Design review of the part shown in the three views and the two pictorial views. Dimensions are in mm from the part's minimum x, y and z. Coordinates: 2 decimals unless noted, no trailing zeros. Loops run counter-clockwise (first coordinate to the right, second up) from the corner with the lowest first, then second, coordinate; pieces in that order, holes last. Notation, with made-up numbers: M 48,18.25 L 90,18.25 A23 ccw 90,34.25 Z; hole C -6.75,-16 d8. An arc over 180 degrees is marked long. Use CSV: the item, a comma, the result in double quotes. Start each with the question number.
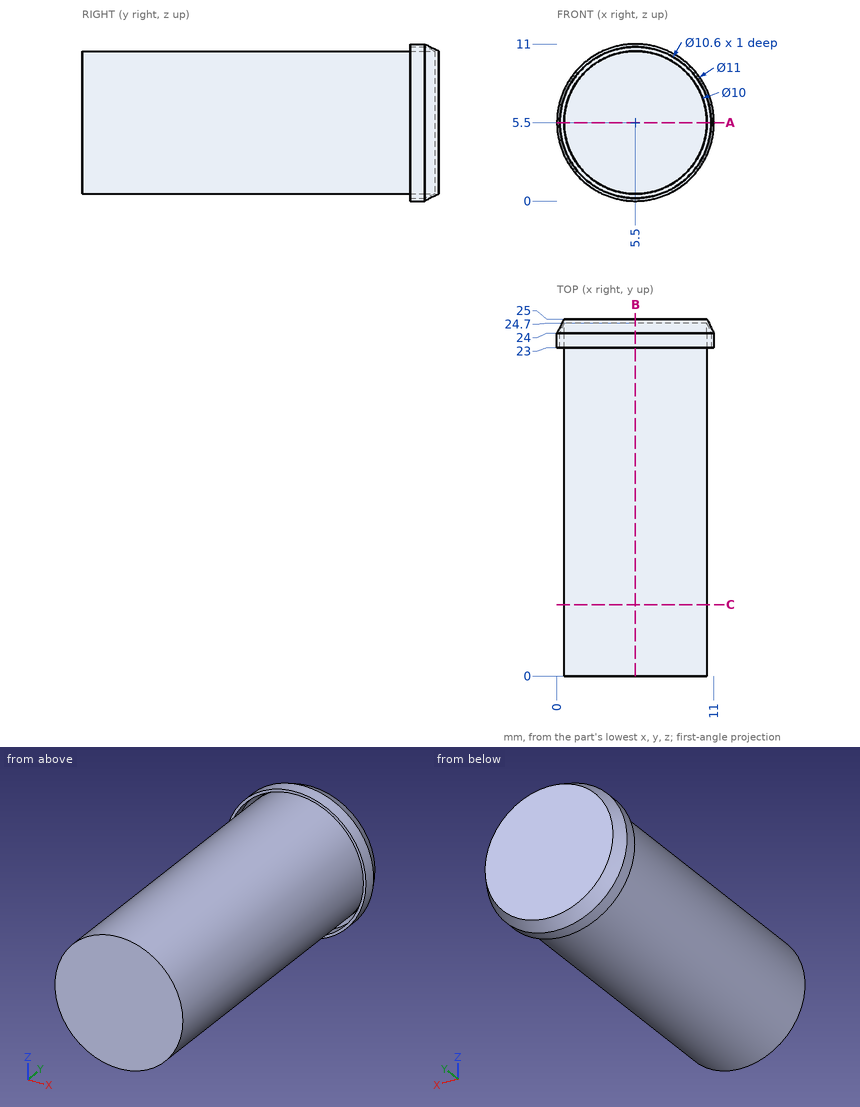
1. Add section B-B (x = 5.5). Write out the cut boundary in (y, z), plus the area to 3 significant figures.
2. Add section A-A (z = 5.5). Write out the cut boundary in (x, y).
3. Add section C-C (y = 5). Write out the cut boundary in (x, z), plus the area to 3 significant figures.
4. To check wall thickness, follow line 1 along Z through (x, y) = (5.5, 23.65); line 2 along X through (y, z) = (23.5, 10); line 3 along Z through (x, y) = (5.75, 18). State the ranges of each line that lie inside material, in increasing order.
5. Insertion check: pin 1 Ø1 at (x, z) = (6.5, 8.5) entering from -Y; pin 2 Ø1.5 at (y, z) = (9.5, 2.5) entering from -X; pin 3 Ø5 at (y, z) = (13.5, 7) entering from -X; pin 4 Ø1 at (y, z) = (6, 4) entering from -X. Each pin has a flat end and moves straight along its axis. Give the tip position at first contact, or say it passes through.
Solved:
1,outline,"M 0,0.5 L 24.7,0.5 L 24,0.2 L 23,0.2 L 23,0 L 24,0 L 25,0.5 L 25,10.5 L 24,11 L 23,11 L 23,10.8 L 24,10.8 L 24.7,10.5 L 0,10.5 Z"
1,area,"251 mm^2"
2,outline,"M 0,23 L 0.2,23 L 0.2,24 L 0.5,24.7 L 0.5,0 L 10.5,0 L 10.5,24.7 L 10.8,24 L 10.8,23 L 11,23 L 11,24 L 10.5,25 L 0.5,25 L 0,24 Z"
3,outline,"C 5.5,5.5 d10"
3,area,"78.5 mm^2"
4,line 1,"z = 0 to 0.2, 0.5 to 10.5, 10.8 to 11"
4,line 2,"x = 2.34 to 2.7, 3.32 to 7.68, 8.3 to 8.66"
4,line 3,"z = 0.51 to 10.49"
5,pin 1,"stops at y = 0"
5,pin 2,"stops at x = 1.03"
5,pin 3,"stops at x = 0.5"
5,pin 4,"stops at x = 0.6"
